The listing builds one solid part. Answer for the finished solid, in the listing's coordinates (mm). Round coordinates to 2 decimals unless told otherwise and drop trailing zeros. Write each loop counter-clockwise with the first axis right and the second up, starting at its lowest first coordinate (ties: lowest second). Pieces come first, ordered by that corner, then holes. Notation, with made-up numbers: (-34.5, 76.5) - (15.5, 76.5) arc R19 cw to (15.5, 103.5) - close; hole circle Ø5 at (-15, -0.75). An arc over 180 degrees is marked (long way). Return JSON: item names as keys, results as strings. Group by question number.
(1) Section D-D, the plane y = 2.75 is taken. Write down the section's boundary in (x, z).
(2) Determine the mould class of faces 1 (the cylindrical face through (-0.596, 2.06, 2.685)), 2 (the flat face through (-3, 0, 0)), 3 (the flat face through (5.08, 2, 0)), 4 (the cylindrical face through (-9.75, 3.03, 0.29)) for opening direction X: +X half, -X half, draft (parallel to the pull), parting line (faces both ways), or undercut.
(3) Find the intervals of material crossed by line 1 along X through (y, z) = (3.05, 0); line 2 along X through (y, z) = (1.05, 0); line 3 along Z through (x, y) = (0, 3.25), in increasing order. Write a range as [from, to].
(4) Section C-C, the plane x = 3.5 is taken. Write down the section's boundary in (y, z).
(5) Each of these flat-tipped pins is pushed along its axis until it touches: pin 1 (1.5 mm diameter, centred on x = -2, y = 1.5, fed in from -Z); pin 2 (1 mm diameter, centred on x = -1.5, y = 1.5, fed in from -Z); pin 3 (1 mm diameter, centred on x = -4.5, z = 9.5, fed in from +Y). Where does it stop, or does it pass through?
(6) Section B-B, the plane x = 0 is taken. Write down the section's boundary in (y, z), then the cut area to 3 significant figures.
(7) Section A-A, the plane z = 0 is taken. Write down the section's boundary in (x, y), then the cut area to 3 significant figures.
Autodesk Inventor part; units mm, degrees
ref_plane "YZ Plane" through (0, 0, 0) normal (1, 0, 0) x (0, 1, 0)
ref_plane "XZ Plane" through (0, 0, 0) normal (0, 1, 0) x (-1, 0, 0)
ref_plane "XY Plane" through (0, 0, 0) normal (0, 0, 1) x (1, 0, 0)
sketch "Sketch1" plane through (0, 0, 0) normal (0, 1, 0) x (-1, 0, 0)
  circle A0 centre (0, 0) radius 11.9126
  dimension "d0" = 23.8252
extrude "Extrusion1" add sketch "Sketch1" along normal blind 2.032
sketch "Sketch2" plane through (0, 2.032, 0) normal (0, 1, 0) x (1, 0, 0)
  circle A0 centre (0, 0) radius 9.7536
  dimension "d3" = 19.5072
extrude "Extrusion2" add sketch "Sketch2" along normal blind 2.032
sketch "Sketch3" plane through (0, 4.064, 0) normal (0, 1, 0) x (1, 0, 0)
  circle A0 centre (0, 0) radius 2.75
  dimension "d6" = 5.5
extrude "Extrusion3" cut sketch "Sketch3" against normal blind 4.064
sketch "Sketch4" plane through (0, 4.064, 0) normal (0, 1, 0) x (1, 0, 0)
  line L0 (17.8511, 14.0442) -> (5.08, 14.0442)
  line L1 (5.08, 14.0442) -> (5.08, -15.9032)
  line L2 (5.08, -15.9032) -> (17.8511, -15.9032)
  line L3 (17.8511, -15.9032) -> (17.8511, 14.0442)
  point P0 (0, 0)
  dimension "d9" = 5.08
extrude "Extrusion4" cut sketch "Sketch4" against normal blind 4.064
properties part number "Spring Clamp Large"
Working result:
{
 "1": {"outline": "(5.08, -8.33) - (5.08, 8.33) arc R9.75 ccw (long way) to start; hole circle Ø5.5 at (0, 0)"},
 "2": {"face 1": "undercut", "face 2": "draft", "face 3": "+X half", "face 4": "parting line"},
 "3": {"line 1": "x = [-9.75, -2.75], [2.75, 5.08]", "line 2": "x = [-11.91, -2.75], [2.75, 5.08]", "line 3": "z = [-9.75, -2.75], [2.75, 9.75]"},
 "4": {"outline": "(0, -11.39) - (2.03, -11.39) - (2.03, -9.1) - (4.06, -9.1) - (4.06, 9.1) - (2.03, 9.1) - (2.03, 11.39) - (0, 11.39) - close"},
 "5": {"pin 1": "stops at z = -11.85", "pin 2": "stops at z = -11.87", "pin 3": "stops at y = 2.03"},
 "6": {"outline": "(0, -11.91) - (2.03, -11.91) - (2.03, -9.75) - (4.06, -9.75) - (4.06, -2.75) - (0, -2.75) - close; (0, 2.75) - (4.06, 2.75) - (4.06, 9.75) - (2.03, 9.75) - (2.03, 11.91) - (0, 11.91) - close", "area": "65.7 mm^2"},
 "7": {"outline": "(-11.91, 0) - (-2.75, 0) - (-2.75, 4.06) - (-9.75, 4.06) - (-9.75, 2.03) - (-11.91, 2.03) - close; (2.75, 0) - (5.08, 0) - (5.08, 4.06) - (2.75, 4.06) - close", "area": "42.3 mm^2"}
}
